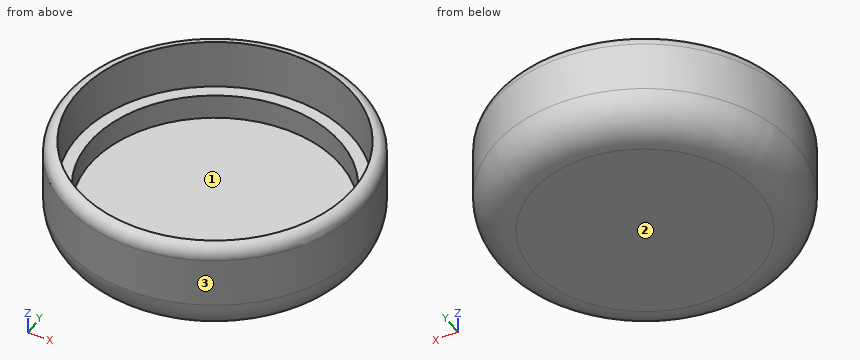
```python
from build123d import *

# Parameters (mm, degrees)
F0_R     = 12
F1_DEPTH = 8
F2_R     = 10
F3_DEPTH = 6
F2_R_2   = 11
F4_DEPTH = 4
F5_R     = 3
F6_R     = 0.99999


# Not quite as in the source:
# - a fillet or chamfer is up to 0.001 mm smaller than in the source, because OpenCascade refuses the exact size


with BuildPart() as f1:
    # F0 (on Top) → F1 (new body)
    with BuildSketch(Plane.XY):
        Circle(F0_R)
    extrude(amount=F1_DEPTH)

    # F2 (on face) → F3 (cut)
    with BuildSketch(Plane.XY.offset(8)):
        Circle(F2_R)
    extrude(amount=-F3_DEPTH, mode=Mode.SUBTRACT)

    # F2 (on face) → F4 (cut)
    with BuildSketch(Plane.XY.offset(8)):
        Circle(F2_R_2)
        Circle(F2_R, mode=Mode.SUBTRACT)
    extrude(amount=-F4_DEPTH, mode=Mode.SUBTRACT)

    # F5
    f5_edges = [f1.edges().sort_by_distance(p)[0] for p in [
        (-12, 0, 0),
    ]]
    fillet(f5_edges, radius=F5_R)

    # F6 (radius 1 in the source; OpenCascade refuses exactly that, so slightly less here)
    f6_edges = [f1.edges().sort_by_distance(p)[0] for p in [
        (-12, 0, 8),
    ]]
    fillet(f6_edges, radius=F6_R)


solid = f1.part
```
The listing builds one solid part. Answer for the finished solid, in the listing's coordinates (mm). Face numbers are marked on the shaded views. Give positions to 0.01 mm unless a question says otherwise; leave off trailing zeros. Order: outer loops, then holes, each group sorted by start corner. A loop starts at its lowest first (then second) coordinate and runs counter-clockwise, first axis right, second up.
Item 1: The part is cut by section C-C, the plane z = 6. Give the vertices of the cut face in (x, y).
From the geometry:
outline: circle Ø24 at (0, 0); hole circle Ø22 at (0, 0)
Item 2: Given pin 1 Ø3 at (x, z) = (-7, 1) entering from -Y; pin 2 Ø1 at (y, z) = (3, 4) entering from +X; pin 3 Ø6 at (x, y) = (-4, -0.5) entering from +Z, each flat-ended and moving along its own axis, determine where each tip first touches the part or whether it passes through.
From the geometry:
pin 1: stops at y = -10.27
pin 2: stops at x = 11.74
pin 3: stops at z = 2
Item 3: The part is cut by section D-D, the plane z = 1.5. Give the vertices of the cut face in (x, y).
From the geometry:
outline: circle Ø23.2 at (0, 0)
Item 4: For a pull along X with two mould halves and no side action, classify the marked faces 1, 2 and 3 as pulls with the +X half, pulls with the -X half, needs draft (parallel to the pull), parting line crosses it, or undercut.
From the geometry:
face 1: undercut
face 2: needs draft
face 3: parting line crosses it
Item 5: Find the intervals of material crossed by probe 1 along Y at (x, z) = (0, 3); probe 2 along Y at (x, z) = (0, 7.1); probe 3 along X at (y, z) = (2.5, 7), in increasing order.
From the geometry:
probe 1: y = -12 to -10, 10 to 12
probe 2: y = -11.99 to -11, 11 to 11.99
probe 3: x = -11.74 to -10.71, 10.71 to 11.74
